from build123d import *

# Parameters (mm, degrees)
SKETCH1_W         = 127
SKETCH1_H         = 76.2
BASE_PLATE_DEPTH  = 9.525
SKETCH2_W         = 38.1
SKETCH2_H         = 38.1
RAISED_BOSS_DEPTH = 6.35
SKETCH3_W         = 12.7
SKETCH3_H         = 25.4
EDGE_NOTCH_DEPTH  = 149.954542143
SKETCH4_R         = 4.7625
HOLE_1_DEPTH      = 149.954542143
SKETCH5_R         = 4.7625
HOLE_2_DEPTH      = 149.954542143
SKETCH6_R         = 4.7625
HOLE_3_DEPTH      = 149.954542143
SKETCH7_R         = 4.7625
HOLE_4_DEPTH      = 149.954542143


with BuildPart() as part:
    # Sketch1 → base_plate (new body)
    with BuildSketch(Plane.XY):
        with Locations((63.5, 38.1)):
            Rectangle(SKETCH1_W, SKETCH1_H)
    extrude(amount=BASE_PLATE_DEPTH)

    # Sketch2 → raised_boss (add)
    with BuildSketch(Plane.XY.offset(9.525)):
        with Locations((63.5, 38.1)):
            Rectangle(SKETCH2_W, SKETCH2_H)
    extrude(amount=RAISED_BOSS_DEPTH)

    # Sketch3 → edge_notch (cut, through all)
    with BuildSketch(Plane.XY):
        with Locations((120.904, 38.1)):
            Rectangle(SKETCH3_W, SKETCH3_H)
    extrude(amount=EDGE_NOTCH_DEPTH, mode=Mode.SUBTRACT)

    # Sketch4 → hole_1 (cut, through all)
    with BuildSketch(Plane.XY):
        with Locations(Location((15.875, 15.875, 0), (0, 0, 180))):
            Circle(SKETCH4_R)
    extrude(amount=HOLE_1_DEPTH, mode=Mode.SUBTRACT)

    # Sketch5 → hole_2 (cut, through all)
    with BuildSketch(Plane.XY):
        with Locations(Location((111.125, 15.875, 0), (0, 0, 180))):
            Circle(SKETCH5_R)
    extrude(amount=HOLE_2_DEPTH, mode=Mode.SUBTRACT)

    # Sketch6 → hole_3 (cut, through all)
    with BuildSketch(Plane.XY):
        with Locations(Location((15.875, 60.325, 0), (0, 0, 180))):
            Circle(SKETCH6_R)
    extrude(amount=HOLE_3_DEPTH, mode=Mode.SUBTRACT)

    # Sketch7 → hole_4 (cut, through all)
    with BuildSketch(Plane.XY):
        with Locations(Location((111.125, 60.325, 0), (0, 0, 180))):
            Circle(SKETCH7_R)
    extrude(amount=HOLE_4_DEPTH, mode=Mode.SUBTRACT)


solid = part.part
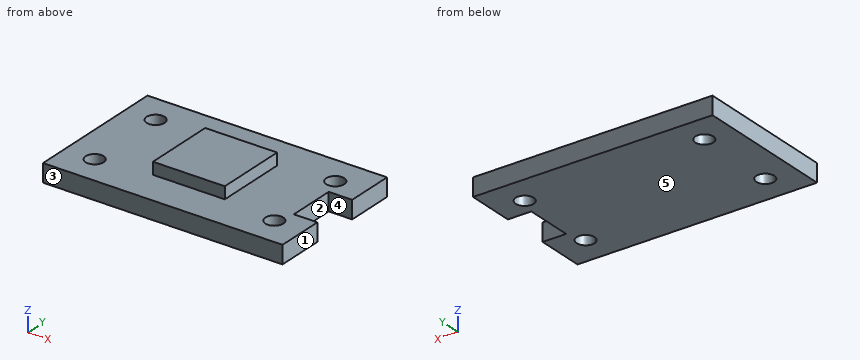
Could you check a few things on this model? Use its own coordinates, in mm. Face numbers are marked on the shaded views. A direction names the side the tool comes from. Coordinates: 2 decimals unless noted, no trailing zeros. Loops run counter-clockwise (first coordinate to the right, second up) from the corner with the lowest first, then second, coordinate; pieces in that order, holes last. Notation, with made-up numbers: (20, -30.5) -> (55, -30.5) arc R18 ccw to (55, -23.5) -> close; hole circle Ø6 at (-37.5, -33.5). An arc over 180 degrees is marked (long way). Answer in a Markdown table with one row per item.
(1) Imagine slicing it at C-C (y = 47). List the corners of the cut face in (x, z) for me (3 decimals), plus the area to 3 significant figures.
Results found:
| item | result |
|---|---|
| outline | (0, 0) -> (114.554, 0) -> (114.554, 9.525) -> (82.55, 9.525) -> (82.55, 15.875) -> (44.45, 15.875) -> (44.45, 9.525) -> (0, 9.525) -> close |
| area | 1,330 mm^2 |
(2) Imagine slicing it at A-A (z = 2). List the corners of the cut face in (x, y) for me (1 decimal), plus the area to 3 significant figures.
Results found:
| item | result |
|---|---|
| outline | (0, 0) -> (127, 0) -> (127, 25.4) -> (114.6, 25.4) -> (114.6, 50.8) -> (127, 50.8) -> (127, 76.2) -> (0, 76.2) -> close; hole circle Ø9.5 at (15.9, 15.9); hole circle Ø9.5 at (15.9, 60.3); hole circle Ø9.5 at (111.1, 15.9); hole circle Ø9.5 at (111.1, 60.3) |
| area | 9,080 mm^2 |
(3) Imagine slicing it at D-D (x = 51.5). List the corners of the cut face in (y, z) for me (3 decimals), plus the area to 3 significant figures.
Results found:
| item | result |
|---|---|
| outline | (0, 0) -> (76.2, 0) -> (76.2, 9.525) -> (57.15, 9.525) -> (57.15, 15.875) -> (19.05, 15.875) -> (19.05, 9.525) -> (0, 9.525) -> close |
| area | 968 mm^2 |
(4) For the marked faces 4 and 5, which set-ups out of +Z, -Z, +X, -X, +Y, -Y let a thin tool reach every point of the face, with its end or its side?
Results found:
| item | result |
|---|---|
| face 4 | +Z, -Z, +X |
| face 5 | -Z, +X, -X, +Y, -Y |
(5) Will these pins go through, and if not, where does the flat tip stop? pin 1 Ø3 at (y, z) = (33, 13.5) entering from +X; pin 2 Ø5 at (x, z) = (62, 14) entering from +Y; pin 3 Ø3 at (y, z) = (32.5, 4) entering from +X.
Results found:
| item | result |
|---|---|
| pin 1 | stops at x = 82.55 |
| pin 2 | stops at y = 57.15 |
| pin 3 | stops at x = 114.55 |
(6) Thinking about a two-plate mould opening in Y: for the marked faces 1, 2 and 3, which applies, released by +Y, released by -Y, zero draft, split by the parting line, or undercut?
Results found:
| item | result |
|---|---|
| face 1 | zero draft |
| face 2 | undercut |
| face 3 | released by -Y |
(7) If I drill on probe 1 along Z at (x, y) = (104, 53.5) (3 decimals); probe 2 along X at (y, z) = (15, 2.75); probe 3 along X at (y, z) = (35.5, 7.25), over which ranges is the centre line in solid material (lowest first)?
Results found:
| item | result |
|---|---|
| probe 1 | z = 0 to 9.525 |
| probe 2 | x = 0 to 11.19, 20.56 to 106.44, 115.81 to 127 |
| probe 3 | x = 0 to 114.55 |
(8) Imagine slicing it at B-B (x = 19). List the corners of the cut face in (y, z) for me (3 decimals), plus the area to 3 significant figures.
Results found:
| item | result |
|---|---|
| outline | (0, 0) -> (12.281, 0) -> (12.281, 9.525) -> (0, 9.525) -> close; (19.469, 0) -> (56.731, 0) -> (56.731, 9.525) -> (19.469, 9.525) -> close; (63.919, 0) -> (76.2, 0) -> (76.2, 9.525) -> (63.919, 9.525) -> close |
| area | 589 mm^2 |
